Could you check a few things on this model? Use its own coordinates, in mm. A direction names the side the tool comes from. Give positions to 0.01 mm unless a question says otherwise; leave off trailing zeros. Order: outer loops, then holes, each group sorted by start corner. A loop starts at its lowest first (then second) coordinate and runs counter-clockwise, first axis right, second up. Notation, with made-up numbers: (-2.5, 31.5) -> (28.5, 31.5) arc R20 cw to (28.5, 66.5) -> close; hole circle Ø6 at (44, -32). An arc over 180 degrees is marked (long way). Write each question's results on one line, items separated by ' | '.
```python
from build123d import *

# Parameters (mm, degrees)
BOSS_EXTRU_1_DEPTH           = 2.5
BOSS_EXTRU_2_DEPTH           = 8.6
ESQUISSE15_W                 = 1.8
ESQUISSE15_H                 = 2.5
D_GAGEMENT_M31_AT_2_COUNT    = 2
D_GAGEMENT_M31_AT_2_PITCH    = 76.2
D_GAGEMENT_M31_AT_3_COUNT    = 2
D_GAGEMENT_M31_AT_3_PITCH    = 38.1
D_GAGEMENT_M31_AT_4_COUNT    = 2
D_GAGEMENT_M31_AT_4_PITCH    = 68.685751798
ESQUISSE16_R                 = 2.7
ENL_V_MAT_EXTRU_2_DEPTH      = 3
ENL_V_MAT_EXTRU_3_DEPTH      = 1.5
ENL_V_MAT_EXTRU_4_DEPTH      = 10
ENL_V_MAT_EXTRU_4_DEPTH_BACK = 10
ESQUISSE20_R                 = 6
CHANFREIN3_SIZE              = 0.577350269
CHANFREIN3_SIZE_2            = 1


with BuildPart() as part:
    # Esquisse1 → Boss.-Extru.1 (new body)
    with BuildSketch(Plane.XY):
        Polygon((0, -85), (17, -102), (121.25, -102), (121.25, 5), (17, 5), (0, -12), align=None)
    extrude(amount=BOSS_EXTRU_1_DEPTH)

    # Esquisse2 → Boss.-Extru.2 (add)
    with BuildSketch(Plane.XY.offset(2.5)):
        Polygon((5, -82.928932188), (19.071067812, -97), (99.25, -97), (99.25, -102), (17, -102), (0, -85), (0, -12), (17, 5), (121.25, 5), (121.25, -102), (106.25, -102), (106.25, -97), (116.25, -97), (116.25, 0), (19.071067812, 0), (5, -14.071067812), align=None)
    extrude(amount=BOSS_EXTRU_2_DEPTH)

    # Esquisse9 → Révolution1 (revolve)
    with BuildSketch(Plane(origin=(0, -55.63, 0), x_dir=(-1, 0, 0), z_dir=(0, -1, 0))):
        Polygon((-96.97, -2.5), (-90.97, -2.5), (-93.47, -4.5), (-96.97, -4.5), align=None)
    revolve(axis=Axis((98.72, -55.63, 2.5), (0, 0, 1)))

    # Esquisse11 → Révolution2 (revolve)
    with BuildSketch(Plane(origin=(0, -55.63, 0), x_dir=(-1, 0, 0), z_dir=(0, -1, 0)), mode=Mode.PRIVATE) as r_volution2_sk:
        Polygon((-24.27, -2.5), (-30.27, -2.5), (-27.77, -4.5), (-24.27, -4.5), align=None)
    revolve(r_volution2_sk.sketch.rotate(Axis((22.52, -55.63, 2.5), (0, 0, 1)), 180), axis=Axis((22.52, -55.63, 2.5), (0, 0, 1)))

    # Esquisse12 → Révolution3 (revolve)
    with BuildSketch(Plane(origin=(0, -17.53, 0), x_dir=(1, 0, 0), z_dir=(0, 1, 0))):
        Polygon((96.97, -2.5), (90.97, -2.5), (93.47, -4.5), (96.97, -4.5), align=None)
    revolve(axis=Axis((98.72, -17.53, 2.5), (0, 0, 1)))

    # Esquisse13 → Révolution4 (revolve)
    with BuildSketch(Plane(origin=(0, -17.53, 0), x_dir=(1, 0, 0), z_dir=(0, 1, 0)), mode=Mode.PRIVATE) as r_volution4_sk:
        Polygon((43.32, -2.5), (49.32, -2.5), (46.82, -4.5), (43.32, -4.5), align=None)
    revolve(r_volution4_sk.sketch.rotate(Axis((41.57, -17.53, 2.5), (0, 0, 1)), 180), axis=Axis((41.57, -17.53, 2.5), (0, 0, 1)))

    # Esquisse15 → Dégagement M31 (revolve, cut)
    with BuildSketch(Plane(origin=(98.72, -55.63, 2.5), x_dir=(0, -1, 0), z_dir=(1, 0, 0))):
        with Locations((0.9, 1.25)):
            Rectangle(ESQUISSE15_W, ESQUISSE15_H)
    d_gagement_m31 = revolve(axis=Axis((98.72, -55.63, 8.85), (0, 0, -1)), mode=Mode.SUBTRACT)

    # Dégagement M31 at 2: Dégagement M31 ×2
    with Locations(*[(-i * D_GAGEMENT_M31_AT_2_PITCH, 0, 0) for i in range(1, D_GAGEMENT_M31_AT_2_COUNT)]):
        add(d_gagement_m31, mode=Mode.SUBTRACT)

    # Dégagement M31 at 3: Dégagement M31 ×2
    with Locations(*[(0, i * D_GAGEMENT_M31_AT_3_PITCH, 0) for i in range(1, D_GAGEMENT_M31_AT_3_COUNT)]):
        add(d_gagement_m31, mode=Mode.SUBTRACT)

    # Dégagement M31 at 4: Dégagement M31 ×2
    with Locations(*[Vector(-0.8320502943378437, 0.5547001962252291, 0) * (i * D_GAGEMENT_M31_AT_4_PITCH) for i in range(1, D_GAGEMENT_M31_AT_4_COUNT)]):
        add(d_gagement_m31, mode=Mode.SUBTRACT)

    # Esquisse16 → Enlèv. mat.-Extru.2 (cut)
    with BuildSketch(Plane(origin=(0, 0, 0), x_dir=(-1, 0, 0), z_dir=(0, 0, -1))):
        with Locations((-22.52, -55.63)):
            Circle(ESQUISSE16_R)
        with Locations((-98.72, -55.63)):
            Circle(ESQUISSE16_R)
        with Locations((-98.72, -17.53)):
            Circle(ESQUISSE16_R)
        with Locations((-41.57, -17.53)):
            Circle(ESQUISSE16_R)
    extrude(amount=-ENL_V_MAT_EXTRU_2_DEPTH, mode=Mode.SUBTRACT)

    # Esquisse17 → Enlèv. mat.-Extru.3 (cut)
    with BuildSketch(Plane.XY.offset(11.1)):
        Polygon((119.75, -99.5), (119.75, 3.5), (17.904163056, 3.5), (1.5, -12.904163056), (1.5, -82.964466094), (18.035533906, -99.5), align=None)
    extrude(amount=-ENL_V_MAT_EXTRU_3_DEPTH, mode=Mode.SUBTRACT)

    # Esquisse20 → Enlèv. mat.-Extru.4 (cut, two sides: drawn at the far end of the back side and taken through both)
    with BuildSketch(Plane.XY.offset(2.5).offset(-ENL_V_MAT_EXTRU_4_DEPTH_BACK)):
        with Locations(Location((98.72, -69.13, 0), (0, 0, 180))):
            Circle(ESQUISSE20_R)
        with Locations(Location((41.52, -69.63, 0), (0, 0, 180))):
            Circle(ESQUISSE20_R)
        with Locations(Location((79.72, -13.03, 0), (0, 0, 180))):
            Circle(ESQUISSE20_R)
    extrude(amount=ENL_V_MAT_EXTRU_4_DEPTH + ENL_V_MAT_EXTRU_4_DEPTH_BACK, mode=Mode.SUBTRACT)

    # Chanfrein3
    # the kernel refuses this chamfer: 1, 0.577350269 mm, written as the material it adds along each edge
    with BuildSketch(Plane(origin=(41.57, -17.53, 3), x_dir=(-1, 0, 0), z_dir=(0, -1, 0))) as chanfrein3_piece_1_section:
        Polygon((2.7, CHANFREIN3_SIZE), (2.7 - CHANFREIN3_SIZE_2, 0), (2.7, 0), align=None)
    chanfrein3_piece_1 = revolve(axis=Axis((41.57, -17.53, 3), (0, 0, -1)), mode=Mode.PRIVATE)
    chanfrein3_piece_1 = chanfrein3_piece_1 - Plane(origin=(41.57, -17.53, 2.701530762), x_dir=(-1, 0, 0), z_dir=(0, 0, -1)) * Cylinder(1.75, 11, mode=Mode.PRIVATE)
    add(chanfrein3_piece_1)
    with BuildSketch(Plane(origin=(98.72, -17.53, 3), x_dir=(-1, 0, 0), z_dir=(0, -1, 0))) as chanfrein3_piece_2_section:
        Polygon((2.7, CHANFREIN3_SIZE), (2.7 - CHANFREIN3_SIZE_2, 0), (2.7, 0), align=None)
    chanfrein3_piece_2 = revolve(axis=Axis((98.72, -17.53, 3), (0, 0, -1)), mode=Mode.PRIVATE)
    chanfrein3_piece_2 = chanfrein3_piece_2 - Plane(origin=(98.72, -17.53, 2.701530762), x_dir=(-1, 0, 0), z_dir=(0, 0, -1)) * Cylinder(1.75, 11, mode=Mode.PRIVATE)
    add(chanfrein3_piece_2)
    with BuildSketch(Plane(origin=(98.72, -55.63, 3), x_dir=(-1, 0, 0), z_dir=(0, -1, 0))) as chanfrein3_piece_3_section:
        Polygon((2.7, CHANFREIN3_SIZE), (2.7 - CHANFREIN3_SIZE_2, 0), (2.7, 0), align=None)
    chanfrein3_piece_3 = revolve(axis=Axis((98.72, -55.63, 3), (0, 0, -1)), mode=Mode.PRIVATE)
    chanfrein3_piece_3 = chanfrein3_piece_3 - Plane(origin=(98.72, -55.63, 2.701530762), x_dir=(-1, 0, 0), z_dir=(0, 0, -1)) * Cylinder(1.75, 11, mode=Mode.PRIVATE)
    add(chanfrein3_piece_3)
    with BuildSketch(Plane(origin=(22.52, -55.63, 3), x_dir=(-1, 0, 0), z_dir=(0, -1, 0))) as chanfrein3_piece_4_section:
        Polygon((2.7, CHANFREIN3_SIZE), (2.7 - CHANFREIN3_SIZE_2, 0), (2.7, 0), align=None)
    chanfrein3_piece_4 = revolve(axis=Axis((22.52, -55.63, 3), (0, 0, -1)), mode=Mode.PRIVATE)
    chanfrein3_piece_4 = chanfrein3_piece_4 - Plane(origin=(22.52, -55.63, 2.701530762), x_dir=(-1, 0, 0), z_dir=(0, 0, -1)) * Cylinder(1.75, 11, mode=Mode.PRIVATE)
    add(chanfrein3_piece_4)


solid = part.part
```
Q1. Thinking about a two-plate mould opening in X: for faces 1 (the flat face through (24, -57, 4.5)), 2 (the flat face through (0, -49, 5)), 3 (the flat face through (68, 5, 5)), which applies, +X half, -X half, draft (parallel to the pull), parting line (faces both ways), or undercut?
Here are the results:
face 1: undercut | face 2: -X half | face 3: draft
Q2. I'm going to push flat-ended pins straight in: pin 1 Ø4 at (x, y) = (22.52, -55.63) entering from -Z; pin 2 Ø4 at (x, y) = (108, -69) entering from +Z; pin 3 Ø4.5 at (x, y) = (98.72, -17.53) entering from -Z. Where does each tip first touch, or does it pass through?
Here are the results:
pin 1: stops at z = 2.83 | pin 2: stops at z = 2.5 | pin 3: stops at z = 2.68
Q3. For faces 4 (the cylindrical face through (22.871, -52.953, 1.194)), 5 (the flat face through (68, -102, 5)), 6 (the flat face through (43, -19, 4.5)), which set-ups out of +Z, -Z, +X, -X, +Y, -Y let a thin tool reach every point of the face, with its end or its side?
Here are the results:
face 4: -Z | face 5: +Z, -Z, +X, -X, -Y | face 6: +Z
Q4. Suppose I cut it at B-B on z = 8.25. Please give me the cut outline in (x, y), and give its area (3 significant figures).
Here are the results:
outline: (0, -85) -> (17, -102) -> (99.25, -102) -> (99.25, -97) -> (19.07, -97) -> (5, -82.93) -> (5, -14.07) -> (19.07, 0) -> (116.25, 0) -> (116.25, -97) -> (106.25, -97) -> (106.25, -102) -> (121.25, -102) -> (121.25, 5) -> (17, 5) -> (0, -12) -> close | area: 2,060 mm²
Q5. Suppose I cut it at D-D on x = 41.57. Please give me the cut outline in (y, z), and give its area (3 significant figures).
Here are the results:
outline: (-102, 0) -> (-75.63, 0) -> (-75.63, 2.5) -> (-97, 2.5) -> (-97, 9.6) -> (-99.5, 9.6) -> (-99.5, 11.1) -> (-102, 11.1) -> close; (-63.63, 0) -> (-20.23, 0) -> (-20.23, 2.42) -> (-19.28, 2.97) -> (-19.28, 4.5) -> (-22.78, 4.5) -> (-25.28, 2.5) -> (-63.63, 2.5) -> close; (-15.78, 2.97) -> (-14.83, 2.42) -> (-14.83, 0) -> (5, 0) -> (5, 11.1) -> (3.5, 11.1) -> (3.5, 9.6) -> (0, 9.6) -> (0, 2.5) -> (-9.78, 2.5) -> (-12.28, 4.5) -> (-15.78, 4.5) -> close | area: 320 mm²
Q6. Suppose I cut it at A-A on x = 22.52. Please give me the cut outline in (y, z), and give its area (3 significant figures).
Here are the results:
outline: (-102, 0) -> (-58.33, 0) -> (-58.33, 2.42) -> (-57.38, 2.97) -> (-57.38, 4.5) -> (-60.88, 4.5) -> (-63.38, 2.5) -> (-97, 2.5) -> (-97, 9.6) -> (-99.5, 9.6) -> (-99.5, 11.1) -> (-102, 11.1) -> close; (-53.88, 2.97) -> (-52.93, 2.42) -> (-52.93, 0) -> (5, 0) -> (5, 11.1) -> (3.5, 11.1) -> (3.5, 9.6) -> (0, 9.6) -> (0, 2.5) -> (-47.88, 2.5) -> (-50.38, 4.5) -> (-53.88, 4.5) -> close | area: 350 mm²
Q7. I need wall thicknesses on line 1 along Y through (x, z) = (98.72, 0.85); line 2 along X through (y, z) = (-14.5, 9); line 3 along Y through (x, z) = (41.57, 1.95). Which ranges of each line are inside material? Lowest first, please.
Here are the results:
line 1: y = -102 to -75.13, -63.13 to -58.33, -52.93 to -20.23, -14.83 to 5 | line 2: x = 0 to 5, 116.25 to 121.25 | line 3: y = -102 to -75.63, -63.63 to -20.23, -14.83 to 5
Q8. Suppose I cut it at C-C on y = -55.63. State how many separate pieces and enclosed holes the cut face has, and give its area (3 significant figures).
Here are the results:
separate pieces: 3 | enclosed holes: 0 | area: 389 mm²
